Part model, mm, in its own coordinate system. Round coordinates to 2 decimals unless told otherwise and drop trailing zeros. Write each loop counter-clockwise with the first axis right and the second up, starting at its lowest first coordinate (ties: lowest second). Pieces come first, ordered by that corner, then holes.
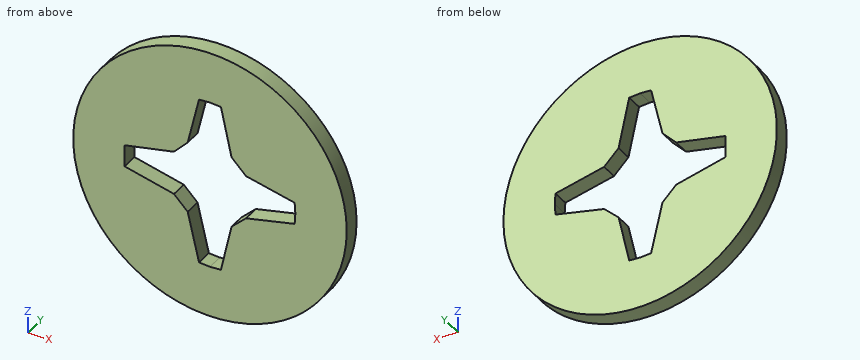
```python
from build123d import *

# Parameters (mm, degrees)
SKETCH1_R           = 24.933599888
BOSS_EXTRUDE1_DEPTH = 3


with BuildPart() as part:
    # Sketch1 → Boss-Extrude1 (new body)
    with BuildSketch(Plane(origin=(0, 0, 0), x_dir=(1, 0, 0), z_dir=(0, 1, 0))):
        with Locations((0.066400112, -0.066400112)):
            Circle(SKETCH1_R)
        Polygon((-15.5, -0.066400112), (-15.5, 1.933599888), (-6.5, 4), (-4, 6.5), (-1.929468724, 15.371518143), (0.066400112, 15.5), (2.058453157, 15.372010982), (4, 6.5), (6.632800224, 4), (15.503783714, 1.933599888), (15.632800224, -0.066400112), (15.503783714, -2.066400112), (6.632800224, -4), (4, -6.632800224), (2.062268949, -15.504318367), (0.066400112, -15.632800224), (-1.929468724, -15.504318367), (-4, -6.632800224), (-6.5, -4), (-15.5, -2.066400112), align=None, mode=Mode.SUBTRACT)
    extrude(amount=BOSS_EXTRUDE1_DEPTH)


solid = part.part
```
Q1. Cut at B-B on x = -8. Write the cut outline in (y, z), plus the area to 3 significant figures.
Values follow:
outline: (0, -23.53) - (3, -23.53) - (3, -3.66) - (0, -3.66) - close; (0, 3.68) - (3, 3.68) - (3, 23.66) - (0, 23.66) - close
area: 120 mm2
Q2. Cut at A-A on y = 1.5. Write the cut outline in (x, z).
Values follow:
outline: circle Ø49.87 at (0.07, 0.07); hole (-15.5, -1.93) - (-6.5, -4) - (-4, -6.5) - (-1.93, -15.37) - (0.07, -15.5) - (2.06, -15.37) - (4, -6.5) - (6.63, -4) - (15.5, -1.93) - (15.63, 0.07) - (15.5, 2.07) - (6.63, 4) - (4, 6.63) - (2.06, 15.5) - (0.07, 15.63) - (-1.93, 15.5) - (-4, 6.63) - (-6.5, 4) - (-15.5, 2.07) - close
Q3. Drop flat-ended pins along their axis: pin 1 (1 mm diameter, centred on x = -6.5, z = 6.5, fed in from -Y); pin 2 (1.5 mm diameter, centred on y = 2, z = 8, fed in from -X). Give the stop position or say it passes through.
Values follow:
pin 1: stops at y = 0
pin 2: stops at x = -23.81
Q4. Cut at C-C on z = 5. Write the cut outline in (x, y), plus the area to 3 significant figures.
Values follow:
outline: (-24.37, 0) - (-5.55, 0) - (-5.55, 3) - (-24.37, 3) - close; (5.63, 0) - (24.51, 0) - (24.51, 3) - (5.63, 3) - close
area: 113 mm2
Q5. Wall check: L1, parallel to X at y = 2, z = -12; L2, parallel to Z at x = 8.5, y = 1.9; L3, parallel to Z at x = 14, y = 2.4. Give the ranges that are in metal, low to high.
Values follow:
L1: x = -21.75 to -2.72, 2.8 to 21.89
L2: z = -23.4 to -3.57, 3.59 to 23.53
L3: z = -20.61 to -2.28, 2.39 to 20.74
Q6. Cut at D-D on x = 18. Write the cut outline in (y, z), plus the area to 3 significant figures.
Values follow:
outline: (0, -17.26) - (3, -17.26) - (3, 17.39) - (0, 17.39) - close
area: 104 mm2
